Input: part model. Units: mm. Frame: model coordinates. Round coordinates to 2 decimals unless told otherwise and drop trailing zeros. Order: outer loops, then holes, each group sorted by start corner. A loop starts at its lowest first (then second) coordinate and runs counter-clockwise, first axis right, second up. Notation, with made-up numbers: M 0,22.25 L 56,22.25 A21 cw 56,55.25 Z; hole C -13,44 d3. An arc over 180 degrees is marked long. One line per question, with ' | ' between items.
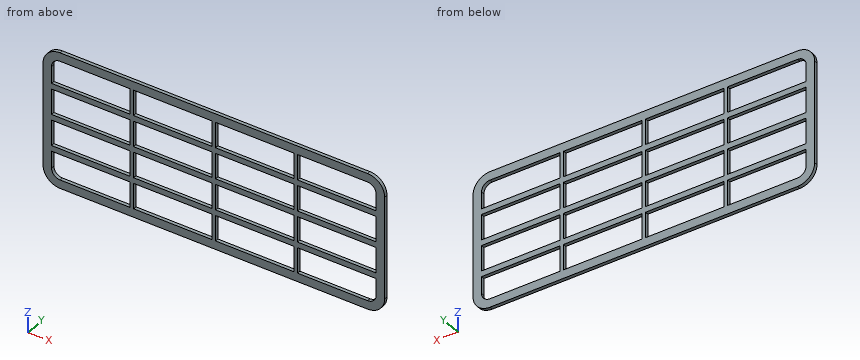
```python
from build123d import *

# Parameters (mm, degrees)
SKETCH1_W           = 23
SKETCH1_H           = 7.5
BOSS_EXTRUDE1_DEPTH = 1


with BuildPart() as part:
    # Sketch1 → Boss-Extrude1 (new body)
    with BuildSketch(Plane(origin=(0, 0, 0), x_dir=(1, 0, 0), z_dir=(0, 1, 0))):
        with BuildLine():
            Line((-68.681780825, 26.812567087), (21.318219175, 26.812567087))
            ThreePointArc((21.318219175, 26.812567087), (24.853753081, 25.348100993), (26.318219175, 21.812567087))
            Line((26.318219175, 21.812567087), (26.318219175, -8.187432913))
            ThreePointArc((26.318219175, -8.187432913), (24.853753081, -11.722966819), (21.318219175, -13.187432913))
            Line((21.318219175, -13.187432913), (-68.681780825, -13.187432913))
            ThreePointArc((-68.681780825, -13.187432913), (-72.217314731, -11.722966819), (-73.681780825, -8.187432913))
            Line((-73.681780825, -8.187432913), (-73.681780825, 21.812567087))
            ThreePointArc((-73.681780825, 21.812567087), (-72.217314731, 25.348100993), (-68.681780825, 26.812567087))
        make_face()
        with BuildLine():
            Line((-71.181780825, 16.812567087), (-48.181780825, 16.812567087))
            Line((-48.181780825, 16.812567087), (-48.181780825, 24.312567087))
            Line((-48.181780825, 24.312567087), (-68.681780825, 24.312567087))
            ThreePointArc((-68.681780825, 24.312567087), (-70.449547778, 23.58033404), (-71.181780825, 21.812567087))
            Line((-71.181780825, 21.812567087), (-71.181780825, 16.812567087))
        make_face(mode=Mode.SUBTRACT)
        with Locations((12.318219175, 11.392567087)):
            Rectangle(SKETCH1_W, SKETCH1_H, mode=Mode.SUBTRACT)
        with BuildLine():
            Line((-71.181780825, -3.187432913), (-48.181780825, -3.187432913))
            Line((-48.181780825, -3.187432913), (-48.181780825, -10.687432913))
            Line((-48.181780825, -10.687432913), (-68.681780825, -10.687432913))
            ThreePointArc((-68.681780825, -10.687432913), (-70.449547778, -9.955199866), (-71.181780825, -8.187432913))
            Line((-71.181780825, -8.187432913), (-71.181780825, -3.187432913))
        make_face(mode=Mode.SUBTRACT)
        with Locations((-35.681780825, 20.562567087)):
            Rectangle(SKETCH1_W, SKETCH1_H, mode=Mode.SUBTRACT)
        with Locations((-11.681780825, 20.562567087)):
            Rectangle(SKETCH1_W, SKETCH1_H, mode=Mode.SUBTRACT)
        with BuildLine():
            Line((0.818219175, 24.312567087), (0.818219175, 16.812567087))
            Line((0.818219175, 16.812567087), (23.818219175, 16.812567087))
            Line((23.818219175, 16.812567087), (23.818219175, 21.812567087))
            ThreePointArc((23.818219175, 21.812567087), (23.085986128, 23.58033404), (21.318219175, 24.312567087))
            Line((21.318219175, 24.312567087), (0.818219175, 24.312567087))
        make_face(mode=Mode.SUBTRACT)
        with Locations((-35.681780825, -6.937432913)):
            Rectangle(SKETCH1_W, SKETCH1_H, mode=Mode.SUBTRACT)
        with Locations((-59.681780825, 11.392567087)):
            Rectangle(SKETCH1_W, SKETCH1_H, mode=Mode.SUBTRACT)
        with Locations((-35.681780825, 11.392567087)):
            Rectangle(SKETCH1_W, SKETCH1_H, mode=Mode.SUBTRACT)
        with Locations((-11.681780825, -6.937432913)):
            Rectangle(SKETCH1_W, SKETCH1_H, mode=Mode.SUBTRACT)
        with BuildLine():
            Line((0.818219175, -10.687432913), (21.318219175, -10.687432913))
            ThreePointArc((21.318219175, -10.687432913), (23.085986128, -9.955199866), (23.818219175, -8.187432913))
            Line((23.818219175, -8.187432913), (23.818219175, -3.187432913))
            Line((23.818219175, -3.187432913), (0.818219175, -3.187432913))
            Line((0.818219175, -3.187432913), (0.818219175, -10.687432913))
        make_face(mode=Mode.SUBTRACT)
        with Locations((-11.681780825, 11.392567087)):
            Rectangle(SKETCH1_W, SKETCH1_H, mode=Mode.SUBTRACT)
        with Locations((-59.681780825, 2.222567087)):
            Rectangle(SKETCH1_W, SKETCH1_H, mode=Mode.SUBTRACT)
        with Locations((-35.681780825, 2.222567087)):
            Rectangle(SKETCH1_W, SKETCH1_H, mode=Mode.SUBTRACT)
        with Locations((-11.681780825, 2.222567087)):
            Rectangle(SKETCH1_W, SKETCH1_H, mode=Mode.SUBTRACT)
        with Locations((12.318219175, 2.222567087)):
            Rectangle(SKETCH1_W, SKETCH1_H, mode=Mode.SUBTRACT)
    extrude(amount=BOSS_EXTRUDE1_DEPTH)


solid = part.part
```
Item 1: Section query C-C, the plane y = 0.25. Give the number of separate pieces and of enclosed holes in the cut face, plus the area to 3 significant figures.
Report:
separate pieces: 1 | enclosed holes: 16 | area: 1,220 mm²
Item 2: Line query: line 1 along Z through (x, y) = (-14, 0.15); line 2 along X through (y, z) = (0.9, -0.5); line 3 along X through (y, z) = (0.15, 9.5). Output: solid intervals per line, ascending. Write a range as from..to.
Report:
line 1: -26.81..-24.31, -16.81..-15.14, -7.64..-5.97, 1.53..3.19, 10.69..13.19 | line 2: -73.68..-71.18, -48.18..-47.18, -24.18..-23.18, -0.18..0.82, 23.82..26.32 | line 3: -73.51..-70.81, -48.18..-47.18, -24.18..-23.18, -0.18..0.82, 23.45..26.14
Item 3: First-contact query: pin 1 (10 mm diameter, centred on x = 0.5, z = -18.5, fed in from -Y). Flat tip, straight axial feed; report the tip coordinate or a pass-through.
Report:
pin 1: y = 0
Item 4: Section query A-A, the plane x = -44. Return loops of the section in (y, z), plus the area to 3 significant figures.
Report:
outline: M 0,-26.81 L 1,-26.81 L 1,-24.31 L 0,-24.31 Z; M 0,-16.81 L 1,-16.81 L 1,-15.14 L 0,-15.14 Z; M 0,-7.64 L 1,-7.64 L 1,-5.97 L 0,-5.97 Z; M 0,1.53 L 1,1.53 L 1,3.19 L 0,3.19 Z; M 0,10.69 L 1,10.69 L 1,13.19 L 0,13.19 Z | area: 10.0 mm²
Item 5: Section query B-B, the plane z = -10. Return loops of the section in (x, y), plus the area to 3 significant figures.
Report:
outline: M -73.68,0 L -71.18,0 L -71.18,1 L -73.68,1 Z; M -48.18,0 L -47.18,0 L -47.18,1 L -48.18,1 Z; M -24.18,0 L -23.18,0 L -23.18,1 L -24.18,1 Z; M -0.18,0 L 0.82,0 L 0.82,1 L -0.18,1 Z; M 23.82,0 L 26.32,0 L 26.32,1 L 23.82,1 Z | area: 8.00 mm²
